Source: CAD feature listing. Evaluate the final solid. Frame: model axes, mm. A direction names the side the tool comes from. Give positions to 0.01 mm unless a question says otherwise; leave off trailing zeros. Order: outer loops, then holes, each group sorted by start corner. A loop starts at its lowest first (then second) coordinate and runs counter-clockwise, first axis right, second up. Notation, with made-up numbers: M 73,-14 L 79,-14 A20 ccw 79,9 Z; hole C -4,49 d4. An arc over 180 degrees is marked long. Answer as a JSON object with one key per item and string values. Group by question number.
1. Section query B-B (x = -38.1). Output: boundary loops of the cut face in (y, z), plus the area to 3 significant figures.
2. Pull-direction query (Y, two-part tool) for faces 1 (the cylindrical face through (41.31, -8.51, 7.4)), 2 (the flat face through (-11.5, -7, 7)), 3 (the flat face through (-6, -12, 46)), 4 (the cylindrical face through (-6.704, -8.635, 66.841)); classes: +Y half, -Y half, draft (parallel to the pull), parting line (faces both ways), or undercut.
3. Section query A-A (z = 5). Output: boundary loops of the cut face in (x, y).
4. Material intervals for L1, parallel to X at y = -9.7, z = 66.25; L2, parallel to X at y = -7.5, z = 7; L3, parallel to Y at x = 15.3, z = 45.85, sorted ascending. Write a range as [from, to].
5. Pin query (flat end, axial travel): P1, Ø4, axis at y = -9.7, z = 58.15, coming from the -X side; P2, Ø3.5, axis at y = -13.5, z = 54, coming from the +X side; P3, Ø4, axis at x = 38.1, y = -7.5, coming from the +Z side; P4, Ø1.4, axis at x = 6.15, y = -9.7, coming from the -Z side. Return the tip coordinate at first contact, or that it passes through.
6. Section query D-D (x = 37.5). Output: boundary loops of the cut face in (y, z), plus the area to 3 significant figures.
7. Section query C-C (z = 58.15). Output: boundary loops of the cut face in (x, y), plus the area to 3 significant figures.
8. Set-up query: faces 5 (the flat face through (14.84, -3.28, 41.11)), 6 (the cylindrical face through (-13.304, -7.395, 1.711)), 7 (the flat face through (0, -9, 65.65)), 8 (the cylindrical face through (-6.26, -13.48, 60.98)), 9 (the flat face through (16, -9, 41)). Return all of +Z, -Z, +X, -X, +Y, -Y with unobstructed straight access to the full face (end or side cutting, diameter ignored); none if empty.
from build123d import *

# Parameters (mm, degrees)
PAD008_DEPTH         = 15
SKETCH021_W          = 27.3
SKETCH021_H          = 27.3
POCKET006_DEPTH      = 12
POCKET007_DEPTH      = 5
SKETCH023_R          = 3.3665
POCKET008_DEPTH      = 68.001
SKETCH024_R          = 1.2
POCKET009_DEPTH      = 2.35
SKETCH026_R          = 1.2
POCKET010_DEPTH      = 33.951
POCKET010_DEPTH_BACK = 61.251
POCKET011_DEPTH      = 63.601


with BuildPart() as part:
    # Sketch020 → Pad008 (new body)
    with BuildSketch(Plane.XZ):
        with BuildLine():
            Line((-47.6, 1.5), (-47.6, 13.5))
            ThreePointArc((-46.1, 15), (-47.1606601718, 14.5606601718), (-47.6, 13.5))
            Line((-46.1, 15), (-23.5, 15))
            ThreePointArc((-23.5, 15), (-18.1966991411, 17.1966991411), (-16, 22.5))
            Line((-16, 22.5), (-16, 68))
            Line((-16, 68), (16, 68))
            Line((16, 68), (16, 22.5))
            ThreePointArc((16, 22.5), (18.1966991411, 17.1966991411), (23.5, 15))
            Line((23.5, 15), (46.1, 15))
            ThreePointArc((47.6, 13.5), (47.1606601718, 14.5606601718), (46.1, 15))
            Line((47.6, 13.5), (47.6, 1.5))
            ThreePointArc((46.1, 0), (47.1606601718, 0.4393398282), (47.6, 1.5))
            Line((46.1, 0), (17.5, 0))
            ThreePointArc((11.5, 6), (13.2573593129, 1.7573593129), (17.5, 0))
            Line((11.5, 9), (11.5, 6))
            ThreePointArc((11.5, 9), (9.7426406871, 13.2426406871), (5.5, 15))
            Line((-5.5, 15), (5.5, 15))
            ThreePointArc((-5.5, 15), (-9.7426406871, 13.2426406871), (-11.5, 9))
            Line((-11.5, 6), (-11.5, 9))
            ThreePointArc((-17.5, 0), (-13.2573593129, 1.7573593129), (-11.5, 6))
            Line((-17.5, 0), (-46.1, 0))
            ThreePointArc((-47.6, 1.5), (-47.1606601718, 0.4393398282), (-46.1, 0))
        make_face()
    extrude(amount=PAD008_DEPTH)

    # Sketch021 (on Face23 of Pad008) → Pocket006 (cut)
    with BuildSketch(Plane(origin=(0, 0, 0), x_dir=(1, 0, 0), z_dir=(0, 1, 0))):
        with Locations((0, -52)):
            Rectangle(SKETCH021_W, SKETCH021_H)
    extrude(amount=-POCKET006_DEPTH, mode=Mode.SUBTRACT)

    # Sketch022 (on Face29 of Pocket006) → Pocket007 (cut)
    with BuildSketch(Plane(origin=(0, -12, 0), x_dir=(1, 0, 0), z_dir=(0, 1, 0))):
        with BuildLine():
            ThreePointArc((-8, -56.0000000001), (-6.2100572838, -61.0433310949), (-1.6412028669, -63.8298437501))
            ThreePointArc((-1.6412028669, -63.8298437501), (0, -65.65), (1.6412028669, -63.8298437501))
            ThreePointArc((1.6412028669, -63.8298437501), (6.2100482063, -61.0433422724), (7.9999999999, -56.0000287985))
            Line((7.9999999999, -56.0000287985), (7.9999999999, -52.0000000001))
            ThreePointArc((8, -52.0000000001), (0, -44.0000000001), (-8, -52.0000000001))
            Line((-8, -52.0000000001), (-8, -56.0000000001))
        make_face()
    extrude(amount=-POCKET007_DEPTH, mode=Mode.SUBTRACT)

    # Sketch023 (on Face22 of Pocket007) → Pocket008 (cut, through all)
    with BuildSketch(Plane(origin=(0, 0, 0), x_dir=(1, 0, 0), z_dir=(0, 0, -1))):
        with Locations((38.1, 7.5)):
            Circle(SKETCH023_R)
        with Locations((-38.1, 7.5)):
            Circle(SKETCH023_R)
    extrude(amount=-POCKET008_DEPTH, mode=Mode.SUBTRACT)

    # Sketch024 (on Face13 of Pocket008) → Pocket009 (cut)
    with BuildSketch(Plane(origin=(0, 0, 68), x_dir=(-1, 0, 0), z_dir=(0, 0, 1))):
        with Locations((-6.15, 9.7)):
            Circle(SKETCH024_R)
        with Locations((6.15, 9.7)):
            Circle(SKETCH024_R)
    extrude(amount=-POCKET009_DEPTH, mode=Mode.SUBTRACT)

    # Sketch026 (on Face27 of Pocket009) → Pocket010 (cut, two sides)
    with BuildSketch(Plane(origin=(-13.65, 0, 0), x_dir=(0, 0, 1), z_dir=(1, 0, 0))) as pocket010_sk:
        with Locations((45.85, 9.7)):
            Circle(SKETCH026_R)
        with Locations((58.15, 9.7)):
            Circle(SKETCH026_R)
    extrude(amount=-POCKET010_DEPTH, mode=Mode.SUBTRACT)
    extrude(pocket010_sk.sketch, amount=POCKET010_DEPTH_BACK, mode=Mode.SUBTRACT)

    # Sketch027 (on Face15 of Pocket010) → Pocket011 (cut, through all)
    with BuildSketch(Plane(origin=(16, 0, 0), x_dir=(0, 0, 1), z_dir=(1, 0, 0))):
        with BuildLine():
            ThreePointArc((66.5, 6.5), (67.5606601718, 6.9393398282), (68, 8))
            Line((68, 8), (68, 0))
            Line((68, 0), (38.35, 0))
            ThreePointArc((38.35, 0), (39.1, 0.2009618943), (39.6490381057, 0.75))
            Line((42.5357894517, 5.75), (39.6490381057, 0.75))
            ThreePointArc((43.8348275573, 6.5), (43.0848275573, 6.2990381057), (42.5357894517, 5.75))
            Line((43.8348275573, 6.5), (66.5, 6.5))
        make_face()
    extrude(amount=-POCKET011_DEPTH, mode=Mode.SUBTRACT)


solid = part.part
Answer sheet:
{
 "1": {"outline": "M -15,0 L -10.87,0 L -10.87,15 L -15,15 Z; M -4.13,0 L 0,0 L 0,15 L -4.13,15 Z", "area": "124 mm^2"},
 "2": {"face 1": "undercut", "face 2": "draft", "face 3": "+Y half", "face 4": "undercut"},
 "3": {"outline": "M -47.6,-15 L -11.58,-15 L -11.58,0 L -47.6,0 Z; M 11.58,-15 L 47.6,-15 L 47.6,0 L 11.58,0 Z; hole C -38.1,-7.5 d6.73; hole C 38.1,-7.5 d6.73"},
 "4": {"L1": "[-16, -7.35], [-4.95, 4.95], [7.35, 16]", "L2": "[-47.6, -41.47], [-34.73, -11.5], [11.5, 34.73], [41.47, 47.6]", "L3": "[-15, -10.9], [-8.5, -6.5]"},
 "5": {"P1": "x = -16", "P2": "x = 16", "P3": "through", "P4": "z = 14.85"},
 "6": {"outline": "M -15,0 L -10.81,0 L -10.81,15 L -15,15 Z; M -4.19,0 L 0,0 L 0,15 L -4.19,15 Z", "area": "126 mm^2"},
 "7": {"outline": "M -16,-15 L -7.71,-15 L -7.71,-12 L -13.65,-12 L -13.65,-10.9 L -16,-10.9 Z; M -16,-8.5 L -13.65,-8.5 L -13.65,-6.5 L -16,-6.5 Z; M 7.71,-15 L 16,-15 L 16,-10.9 L 13.65,-10.9 L 13.65,-12 L 7.71,-12 Z; M 13.65,-8.5 L 16,-8.5 L 16,-6.5 L 13.65,-6.5 Z", "area": "64.3 mm^2"},
 "8": {"face 5": "+Z, +X, -X, +Y", "face 6": "-Z, +Y, -Y", "face 7": "+Y", "face 8": "+Y, -Y", "face 9": "+Z, +X, +Y, -Y"}
}
